Geometry: see drawing. Coordinates: mm, zero at the bounding-box minimum. Round coordinates to 2 decimals unless told otherwise and drop trailing zeros. Order: outer loops, then holes, each group sorted by start corner. A loop starts at its lowest first (then second) coordinate and runs counter-clockwise, first axis right, second up. Notation, with made-up numbers: (62.25, -35) -> (76.25, -35) arc R28 ccw to (76.25, -1) -> close; hole circle Ø9 at (12.25, 44). An arc over 180 degrees is marked (long way). Use a Markdown table: item, result.
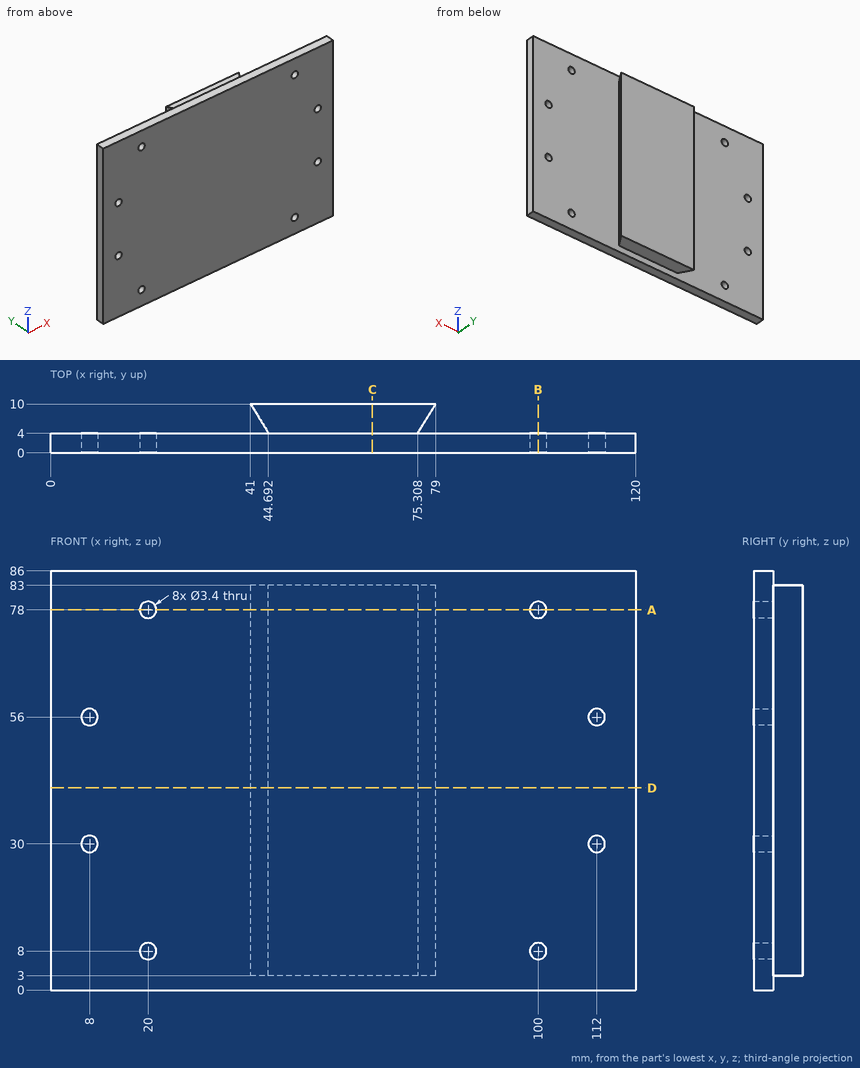
1) Cut plane A-A on z = 78. Return loops of the section in (x, y).
Answer key:
| item | result |
|---|---|
| outline | (0, 0) -> (18.3, 0) -> (18.3, 4) -> (0, 4) -> close; (21.7, 0) -> (98.3, 0) -> (98.3, 4) -> (75.31, 4) -> (79, 10) -> (41, 10) -> (44.69, 4) -> (21.7, 4) -> close; (101.7, 0) -> (120, 0) -> (120, 4) -> (101.7, 4) -> close |
2) Cut plane D-D on z = 41.5. Return loops of the section in (x, y).
Answer key:
| item | result |
|---|---|
| outline | (0, 0) -> (120, 0) -> (120, 4) -> (75.31, 4) -> (79, 10) -> (41, 10) -> (44.69, 4) -> (0, 4) -> close |
3) Cut plane C-C on x = 66. Return loops of the section in (y, z), and give its area (3 significant figures).
Answer key:
| item | result |
|---|---|
| outline | (0, 0) -> (4, 0) -> (4, 3) -> (10, 3) -> (10, 83) -> (4, 83) -> (4, 86) -> (0, 86) -> close |
| area | 824 mm^2 |
4) Contact query for flat-ended pins moving along their axis: P1, Ø5.5, axis at x = 100, z = 8, coming from the +Y side; P2, Ø2, axis at y = 2, z = 39.5, coming from the -X side; P3, Ø5, axis at x = 56.5, y = 7, coming from the +Z side; P4, Ø5, axis at y = 8, z = 38, coming from the +X side. Output: stop coordinate, or through.
Answer key:
| item | result |
|---|---|
| P1 | stops at y = 4 |
| P2 | stops at x = 0 |
| P3 | stops at z = 83 |
| P4 | stops at x = 79 |
5) Ray query, probe 1 along X at (y, z) = (2.5, 30); probe 2 along Z at (x, y) = (20, 2.4); probe 3 along Y at (x, z) = (19.5, 67). Return the intervals inside material, ascending.
Answer key:
| item | result |
|---|---|
| probe 1 | x = 0 to 6.3, 9.7 to 110.3, 113.7 to 120 |
| probe 2 | z = 0 to 6.3, 9.7 to 76.3, 79.7 to 86 |
| probe 3 | y = 0 to 4 |
6) Cut plane B-B on x = 100. Return loops of the section in (y, z), and give its area (3 significant figures).
Answer key:
| item | result |
|---|---|
| outline | (0, 0) -> (4, 0) -> (4, 6.3) -> (0, 6.3) -> close; (0, 9.7) -> (4, 9.7) -> (4, 76.3) -> (0, 76.3) -> close; (0, 79.7) -> (4, 79.7) -> (4, 86) -> (0, 86) -> close |
| area | 317 mm^2 |
